Input: part model. Units: mm. Frame: model coordinates. Face numbers are marked on the shaded views. A direction names the side the tool comes from. Give positions to 0.01 mm unless a question says otherwise; leave off trailing zeros. Write each loop counter-clockwise with the first axis right and the second up, starting at its lowest first coordinate (ties: lowest second). Pieces come first, ordered by that corner, then holes. Notation, with made-up numbers: (-20.5, 4) - (30.5, 4) arc R17 ccw to (30.5, 33) - close; hole circle Ø2 at (1, -25). An arc over 180 degrees is marked (long way). Answer as a JSON object with one key per item and string values. Group by question number.
from build123d import *

# Parameters (mm, degrees)
SKETCH_1_R               = 12
SKETCH_1_R_2             = 9
EXTRUDE_1_DEPTH          = 50
SKETCH_2_R               = 1.65
EXTRUDE_2_DEPTH          = 3
SKETCH_3_R               = 1.75
CUT_EXTRUDE_1_DEPTH      = 13
CUT_EXTRUDE_1_DEPTH_BACK = 13
MIRROR_2_COPY_1_SKETCH_R = 1.65
MIRROR_2_COPY_1_DEPTH    = 3
SKETCH_5_R               = 1.65
EXTRUDE_3_DEPTH          = 3
SKETCH_6_R               = 2.5
EXTRUDE_4_DEPTH          = 2.5


with BuildPart() as part:
    # ｽｹｯﾁ1 → ﾎﾞｽ - 押し出し1 (new body)
    with BuildSketch(Plane.XY):
        Circle(SKETCH_1_R)
        Circle(SKETCH_1_R_2, mode=Mode.SUBTRACT)
    extrude(amount=EXTRUDE_1_DEPTH)

    # ｽｹｯﾁ2 → ﾎﾞｽ - 押し出し2 (add)
    with BuildSketch(Plane(origin=(3, 0, 0), x_dir=(0, 0, -1), z_dir=(1, 0, 0))):
        with BuildLine():
            Line((-43, 9), (-43, 14))
            Line((-43, 14), (-37.994493332, 19.651982218))
            ThreePointArc((-37.994493332, 19.651982218), (-35, 21), (-32.005506668, 19.651982218))
            Line((-32.005506668, 19.651982218), (-27, 14))
            Line((-27, 14), (-27, 9))
            Line((-27, 9), (-43, 9))
        make_face()
        with Locations((-35, 17)):
            Circle(SKETCH_2_R, mode=Mode.SUBTRACT)
    extrude_2 = extrude(amount=EXTRUDE_2_DEPTH)

    # ﾐﾗｰ1: ﾎﾞｽ - 押し出し2 across plane
    add(extrude_2.mirror(Plane(origin=(0, 0, 0), x_dir=(0, 0, 1), z_dir=(1, 0, 0))))

    # ｽｹｯﾁ3 → ｶｯﾄ - 押し出し1 (cut, two sides)
    with BuildSketch(Plane(origin=(0, 0, 0), x_dir=(0, 0, -1), z_dir=(1, 0, 0))) as cut_extrude_1_sk:
        with Locations((-25, 0)):
            Circle(SKETCH_3_R)
    extrude(amount=CUT_EXTRUDE_1_DEPTH, mode=Mode.SUBTRACT)
    extrude(cut_extrude_1_sk.sketch, amount=-CUT_EXTRUDE_1_DEPTH_BACK, mode=Mode.SUBTRACT)

    # ﾐﾗｰ2: ﾎﾞｽ - 押し出し2 across plane
    add(extrude_2.mirror(Plane.ZX))

    # ﾐﾗｰ2 copy 1 sketch → ﾐﾗｰ2 copy 1 (add)
    with BuildSketch(Plane(origin=(-3, 0, 0), x_dir=(0, 0, -1), z_dir=(-1, 0, 0))):
        with BuildLine():
            Line((-43, 9), (-43, 14))
            Line((-43, 14), (-37.994493332, 19.651982218))
            ThreePointArc((-37.994493332, 19.651982218), (-35, 21), (-32.005506668, 19.651982218))
            Line((-32.005506668, 19.651982218), (-27, 14))
            Line((-27, 14), (-27, 9))
            Line((-27, 9), (-43, 9))
        make_face()
        with Locations((-35, 17)):
            Circle(MIRROR_2_COPY_1_SKETCH_R, mode=Mode.SUBTRACT)
    extrude(amount=MIRROR_2_COPY_1_DEPTH)

    # ｽｹｯﾁ5 → ﾎﾞｽ - 押し出し3 (add)
    with BuildSketch(Plane(origin=(0, 3, 0), x_dir=(1, 0, 0), z_dir=(0, 1, 0))):
        with BuildLine():
            Line((9, -7), (14, -7))
            Line((14, -7), (19.651982218, -12.005506668))
            ThreePointArc((19.651982218, -12.005506668), (21, -15), (19.651982218, -17.994493332))
            Line((19.651982218, -17.994493332), (14, -23))
            Line((14, -23), (9, -23))
            Line((9, -23), (9, -7))
        make_face()
        with Locations((17, -15)):
            Circle(SKETCH_5_R, mode=Mode.SUBTRACT)
    extrude_3 = extrude(amount=EXTRUDE_3_DEPTH)

    # ﾐﾗｰ3: ﾎﾞｽ - 押し出し3 across plane
    add(extrude_3.mirror(Plane.ZX))

    # ｽｹｯﾁ6 → ﾎﾞｽ - 押し出し4 (add, symmetric)
    with BuildSketch(Plane(origin=(0, 0, 35), x_dir=(-1, 0, 0), z_dir=(0, 0, -1))):
        with BuildLine():
            Line((-6.095653088, 10.336489415), (-9.685560651, 13.348779527))
            ThreePointArc((-9.685560651, 13.348779527), (-15.320888862, 12.855752194), (-14.827861529, 7.220423983))
            Line((-14.827861529, 7.220423983), (-11.237953965, 4.20813387))
            Line((-11.237953965, 4.20813387), (-6.095653088, 10.336489415))
        make_face()
        with Locations((-12.25671109, 10.284601755)):
            Circle(SKETCH_6_R, mode=Mode.SUBTRACT)
    extrude_4 = extrude(amount=EXTRUDE_4_DEPTH, both=True)

    # ﾐﾗｰ4: ﾎﾞｽ - 押し出し4 across plane
    add(extrude_4.mirror(Plane.ZX))


solid = part.part
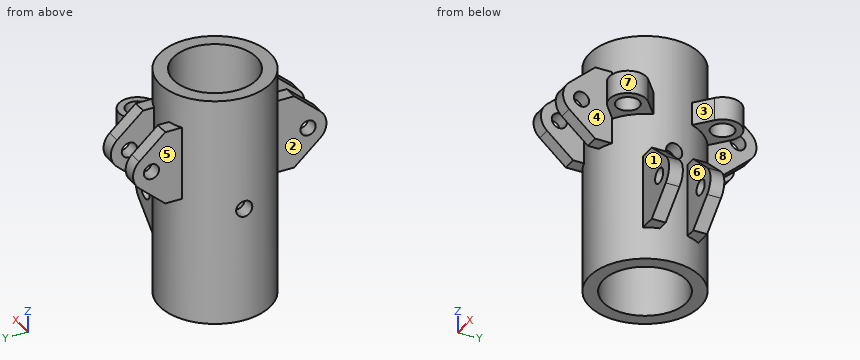
1) Cut plane D-D on z = 40. Return the cut outline in (x, y), and give its area (3 significant figures).
2) Cut plane C-C on y = 0. Return the cut outline in (x, z).
3) Mould query, pull axis X, two halves, no side actions, for the marked faces 5, 6, 7 and 8. Classes: +X half, -X half, draft (parallel to the pull), parting line (faces both ways), or undercut.
4) Cut plane A-A on z = 15. Return the cut outline in (x, y).
5) Reachability of the marked faces 1, 2, 3 and 4 from +Z, -Z, +X, -X, +Y, -Y: full face, straight path, thin tool, end or side. Return the list, or none.
6) Pin query (flat end, axial travel): P1, Ø1.5, axis at y = -13.5, z = 19, coming from the -X side; P2, Ø1.5, axis at x = 6, y = 16, coming from the +Z side; P3, Ø0.9, axis at x = 12.5, y = -4, coming from the +Z side; P4, Ø1, axis at y = -8.5, z = 32.5, coming from the +X side. Return the tip coordinate at first contact, or that it passes through.
7) Cut plane B-B on x = 0. Return the cut outline in (y, z), and give its area (3 significant figures).
8) Line query: line 1 along Y through (x, z) = (5.5, 34.5); line 2 along Z through (x, y) = (10.65, 0); line 3 along X through (y, z) = (0, 39). Output: solid intervals per line, ascending. Write a range as from..to.
Filled in:
{
 "1": {"outline": "(-6, -17.39) - (-3, -17.39) - (-3, -11.62) arc R12 ccw to (3, -11.62) - (3, -17.39) - (6, -17.39) - (6, -10.39) arc R12 ccw to (6, 10.39) - (6, 17.39) - (3, 17.39) - (3, 11.62) arc R12 ccw to (-3, 11.62) - (-3, 17.39) - (-6, 17.39) - (-6, 10.39) arc R12 ccw to (-6, -10.39) - close; hole circle Ø18 at (0, 0)", "area": "274 mm²"},
 "2": {"outline": "(-12, 0) - (-9, 0) - (-9, 23.25) - (-12, 23.25) - close; (-12, 26.75) - (-9, 26.75) - (-9, 50) - (-12, 50) - close; (9, 0) - (12, 0) - (12, 23.25) - (9, 23.25) - close; (9, 26.75) - (12, 26.75) - (12, 50) - (9, 50) - close"},
 "3": {"face 5": "-X half", "face 6": "draft", "face 7": "undercut", "face 8": "undercut"},
 "4": {"outline": "(10.39, -6) - (15.35, -6) - (15.35, -3) - (11.62, -3) arc R12 ccw to (11.62, 3) - (15.35, 3) - (15.35, 6) - (10.39, 6) arc R12 ccw (long way) to start; (18.65, -6) - (21, -6) - (21, -3) - (18.65, -3) - close; (18.65, 3) - (21, 3) - (21, 6) - (18.65, 6) - close; hole circle Ø18 at (0, 0)"},
 "5": {"face 1": "-Z, +X, -Y", "face 2": "+Z, -Z, -X, -Y", "face 3": "+Z, +X", "face 4": "+Z, -Z, -Y"},
 "6": {"P1": "passes through", "P2": "stops at z = 41.89", "P3": "stops at z = 23", "P4": "stops at x = 16.04"},
 "7": {"outline": "(-12, 0) - (-9, 0) - (-9, 50) - (-12, 50) - close; (9, 0) - (12, 0) - (12, 50) - (9, 50) - close", "area": "300 mm²"},
 "8": {"line 1": "y = -20.97..-18.57, -15.43..-7.12, 7.12..15.43, 18.57..20.97", "line 2": "z = 0..23.25, 26.75..50", "line 3": "x = -12..-9, 9..12"}
}
